Can you work these out from the model? Positions are in its coordinate system, mm. Face numbers are marked on the shaded views. Give positions to 0.01 mm unless a question says otherwise; leave off trailing zeros. Order: outer loops, then holes, each group sorted by start corner. A loop starts at its lowest first (then second) coordinate and runs counter-clockwise, first axis right, second up. Notation, with made-up numbers: M 15.5,80.5 L 52.5,80.5 A23 ccw 52.5,106.5 Z; hole C 58,-37 d8. An arc over 180 degrees is marked long. One line per question, with ' | ' between items. Start each with the question number.
1) If we section it at B-B, the plane z = 10.5: Please give me the cut outline in (x, y).
2) Please list where these lines run through material, in increasing order: line 1 along Y through (x, z) = (0, 10.5); line 2 along Y through (x, z) = (0, -23.5); line 3 along X through (y, z) = (-4, 1.5). Write a range as [from, to].
3) If we section it at C-C, the plane z = -20: Please give me the cut outline in (x, y).
4) If we section it at A-A, the plane x = 0: Please give me the cut outline in (y, z).
5) Thinking about a two-plate mould opening in Y: for the marked faces 1 and 2, which applies, +Y half, -Y half, draft (parallel to the pull), parting line (faces both ways), or undercut?
6) I'm going to push flat-ended pins straight in: pin 1 Ø4 at (y, z) = (0, -16) entering from +X; pin 2 Ø1.5 at (y, z) = (6, 25) entering from -X; pin 3 Ø9 at (x, y) = (0, 0) entering from +Z; pin 4 Ø6 at (x, y) = (3, 0) entering from +Z. Where does each tip first touch, or does it pass through?
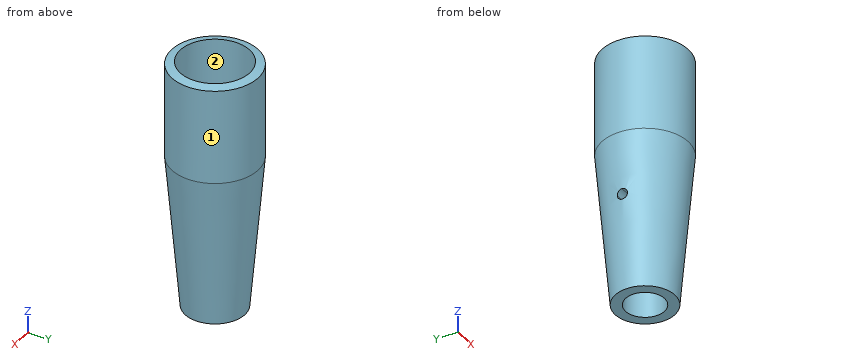
```python
from build123d import *

# Parameters (mm, degrees)
F0_R     = 10.25
F0_R_2   = 5.75
F1_DEPTH = 20
F0_R_3   = 12.75
F2_DEPTH = 35
F3_DEPTH = 40
F5_SIZE2 = 3.9369898587
F5_SIZE  = 45
F7_DEPTH = 25


# Not quite as in the source:
# - a fillet or chamfer that OpenCascade refuses, or shapes differently, is made with other operations: its cross-section is extruded or revolved along the edge and cut away or added


with BuildPart() as f1:
    # F0 (on Top) → F1 (new body)
    with BuildSketch(Plane.XY):
        Circle(F0_R)
        Circle(F0_R_2, mode=Mode.SUBTRACT)
    extrude(amount=F1_DEPTH)

    # F0 (on Top) → F2 (join)
    with BuildSketch(Plane.XY):
        Circle(F0_R_3)
        Circle(F0_R, mode=Mode.SUBTRACT)
    extrude(amount=F2_DEPTH)

    # F3 (add): a face of the model
    f3_faces = [f1.faces().sort_by_distance(p)[0] for p in [
        (-6.1106244584, 0, 0),
    ]]
    extrude(f3_faces, amount=F3_DEPTH)

    # F4: chamfer of 8 x 2.1435935394 on 1 edges, made by hand

    # F4_s1 → F4_t2 (revolve, cut)
    with BuildSketch(Plane.XZ):
        Polygon((12.75, 32.8564064606), (4.75, 35), (12.75, 35), align=None)
    revolve(axis=Axis((0, 0, 35), (0, 0, 1)), mode=Mode.SUBTRACT)

    # F5
    f5_edges = [f1.edges().sort_by_distance(p)[0] for p in [
        (-12.75, 0, -40),
    ]]
    f5_side = f1.faces().sort_by_distance((-12.75, 0, -3.571797))[0]
    chamfer(f5_edges, length=F5_SIZE, length2=F5_SIZE2, reference=f5_side)

    # F6 (on Right) → F7 (cut)
    with BuildSketch(Plane.YZ):
        with BuildLine():
            ThreePointArc((0, -11.2528902143), (-1.5, -12.7528902143), (0, -14.2528902143))
            Line((0, -14.2528902143), (0, -11.2528902143))
        make_face()
        with BuildLine():
            Line((0, -11.2528902143), (0, -14.2528902143))
            ThreePointArc((0, -14.2528902143), (1.0606601718, -13.8135503861), (1.5, -12.7528902143))
            ThreePointArc((1.5, -12.7528902143), (1.0606601718, -11.6922300425), (0, -11.2528902143))
        make_face()
    extrude(amount=-F7_DEPTH, mode=Mode.SUBTRACT)


solid = f1.part
```
Results found:
1) outline: C 0,0 d25.5; hole C 0,0 d11.5
2) line 1: y = [-12.75, -5.75], [5.75, 12.75] | line 2: y = [-10.26, -5.75], [5.75, 10.26] | line 3: x = [-11.78, -4.13], [4.13, 11.78]
3) outline: C 0,0 d21.13; hole C 0,0 d11.5
4) outline: M -12.75,5 L -8.81,-40 L -5.75,-40 L -5.75,20 L -10.25,20 L -10.25,33.53 L -12.75,32.86 Z; M 5.75,-40 L 8.81,-40 L 12.75,5 L 12.75,32.86 L 10.25,33.53 L 10.25,20 L 5.75,20 Z
5) face 1: parting line | face 2: undercut
6) pin 1: stops at x = 11.09 | pin 2: stops at x = -11.62 | pin 3: passes through | pin 4: stops at z = 20
